Can you work these out from the drawing? Everything is in mm from the part's minimum corner. A direction names the side the tool comes from. Coordinates: 2 decimals unless noted, no trailing zeros. Loops run counter-clockwise (first coordinate to the right, second up) from the corner with the lowest first, then second, coordinate; pieces in that order, holes last.
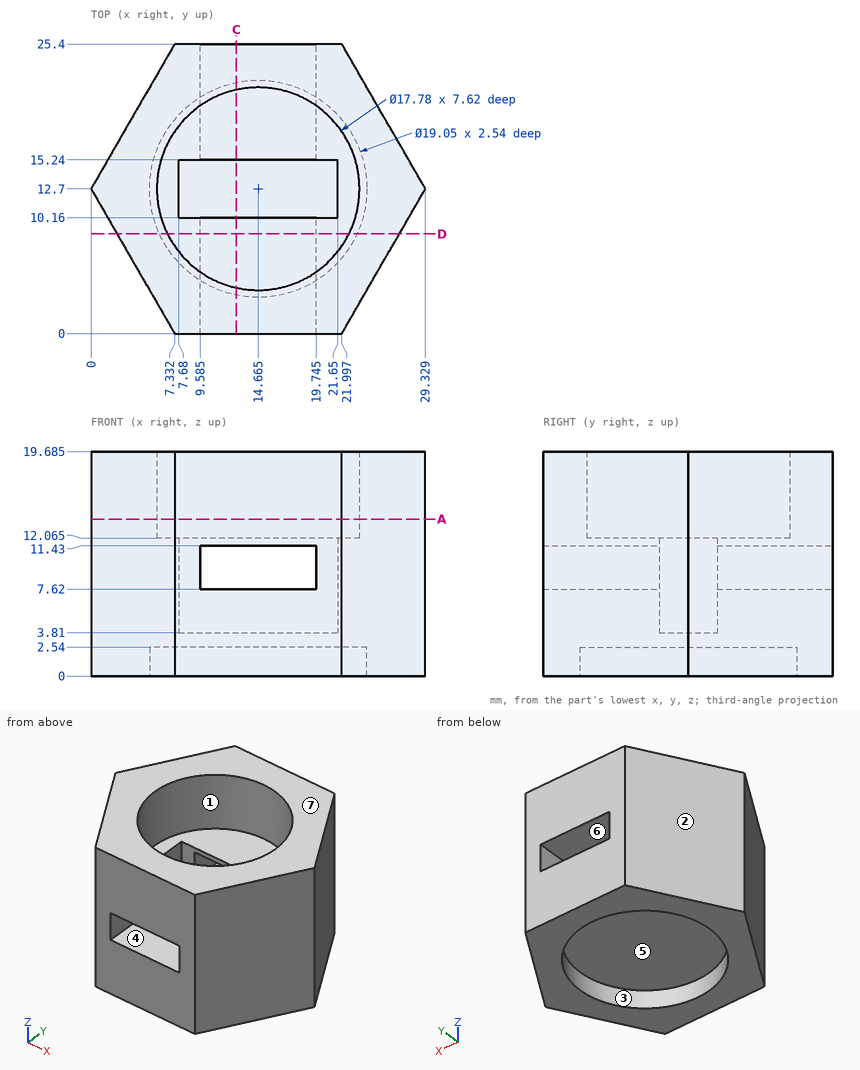
(1) For pin 1 (6 mm diameter, centred on x = 3, z = 11, fed in from +Y); pin 2 (1 mm diameter, centred on y = 15, z = 13, fed in from +X); pin 3 (1.1 mm diameter, centred on y = 21.5, z = 9, fed in from +X), each with a flat end and sliding along its axis, tell me the tip position at first contact or that it passes through.
Answers:
pin 1: stops at y = 23.09
pin 2: stops at x = 28.29
pin 3: stops at x = 24.57
(2) Imagine slicing it at D-D, the plane y = 8.75. Write out the boundary of the cut face in (x, z) (1 decimal).
Answers:
outline: (2.3, 0) - (6, 0) - (6, 2.5) - (23.3, 2.5) - (23.3, 0) - (27, 0) - (27, 19.7) - (22.6, 19.7) - (22.6, 12.1) - (6.7, 12.1) - (6.7, 19.7) - (2.3, 19.7) - close; hole (9.6, 7.6) - (19.7, 7.6) - (19.7, 11.4) - (9.6, 11.4) - close
(3) Which directions (+Z, -Z, +X, -X, +Y, -Y) give clear straight access to the entire face, cutting with the end or side of a thin tool? Please do the marked faces 1, 2 and 3.
Answers:
face 1: +Z
face 2: +Z, -Z, -X, +Y
face 3: -Z
(4) We'd pull the mould along Z, two halves only. Please class the marked faces 4, 5, 6 and 7: +Z half, -Z half, draft (parallel to the pull), parting line (faces both ways), or undercut.
Answers:
face 4: undercut
face 5: -Z half
face 6: undercut
face 7: +Z half
(5) Imagine slicing it at A-A, the plane z = 13.75. Write out the boundary of the cut face in (x, y) (1 decimal).
Answers:
outline: (0, 12.7) - (7.3, 0) - (22, 0) - (29.3, 12.7) - (22, 25.4) - (7.3, 25.4) - close; hole circle Ø17.8 at (14.7, 12.7)
(6) I need wall thicknesses on probe 1 along Z at (x, y) = (17.5, 9.75) (1 decimal); probe 2 along Y at (x, z) = (20.5, 8); probe 3 along Y at (x, z) = (7.25, 13) (1 decimal). Which ranges of each line are inside material? Lowest first, please.
Answers:
probe 1: z = 2.5 to 7.6, 11.4 to 12.1
probe 2: y = 0 to 10.16, 15.24 to 25.4
probe 3: y = 0.1 to 7.8, 17.6 to 25.3
(7) Imagine slicing it at C-C, the plane x = 12.75. Write out the boundary of the cut face in (y, z) (1 decimal).
Answers:
outline: (0, 0) - (3.4, 0) - (3.4, 2.5) - (22, 2.5) - (22, 0) - (25.4, 0) - (25.4, 7.6) - (15.2, 7.6) - (15.2, 3.8) - (10.2, 3.8) - (10.2, 7.6) - (0, 7.6) - close; (0, 11.4) - (10.2, 11.4) - (10.2, 12.1) - (4, 12.1) - (4, 19.7) - (0, 19.7) - close; (15.2, 11.4) - (25.4, 11.4) - (25.4, 19.7) - (21.4, 19.7) - (21.4, 12.1) - (15.2, 12.1) - close
